Study the drawing (mm; zero at the part's minimum x, y, z) and answer. Round coordinates to 2 decimals unless told otherwise and drop trailing zeros. Order: outer loops, then holes, each group sorted by start corner. A loop starts at its lowest first (then second) coordinate and runs counter-clockwise, first axis right, second up. Notation, with made-up numbers: (-4, -18.75) - (5, -18.75) arc R32 ccw to (5, 7.25) - close; hole circle Ø10 at (-23, 70). An arc over 180 degrees is marked (long way). Use one line per item in the form item = value. Start each with the question number.
Q1. The part is cut by section B-B on y = 0.6. Determine the outline of the cut face in (x, z) (1 decimal).
Q2. The part is cut by section D-D on z = 14. Determine the outline of the cut face in (x, y) (1 decimal).
Q3. The part is cut by section C-C on x = 62.5. Determine the outline of the cut face in (y, z), plus the area to 3 significant figures.
Q4. Find the intervals of material crossed by line 1 (Z direction, x = 41, y = 0.9); line 2 (X direction, y = 1.7, z = 30) (1 decimal); line 3 (X direction, y = 0.45, z = 26) (1 decimal), in increasing order. Write a range as [from, to].
Q5. The part is cut by section A-A on z = 32.5. Determine the outline of the cut face in (x, y) (1 decimal), plus the area to 3 significant figures.
Q6. Given P1, Ø1, axis at y = 1, z = 20.5, coming from the +X side (1 decimal), flat-ended and moving along its own axis, determine where the tip first touches the part or whether it passes through.
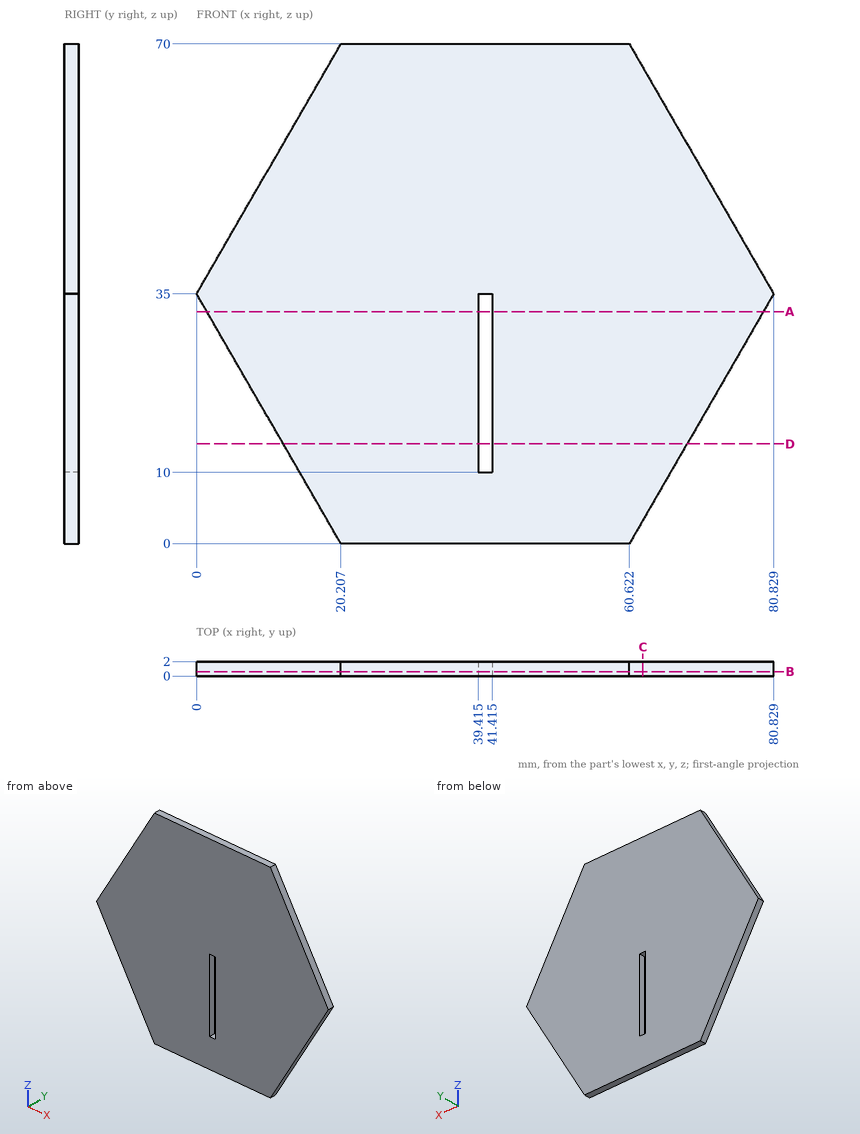
Found:
q1.outline = (0, 35) - (20.2, 0) - (60.6, 0) - (80.8, 35) - (60.6, 70) - (20.2, 70) - close; hole (39.4, 10) - (41.4, 10) - (41.4, 35) - (39.4, 35) - close
q2.outline = (12.1, 0) - (39.4, 0) - (39.4, 2) - (12.1, 2) - close; (41.4, 0) - (68.7, 0) - (68.7, 2) - (41.4, 2) - close
q3.outline = (0, 3.25) - (2, 3.25) - (2, 66.75) - (0, 66.75) - close
q3.area = 127 mm²
q4.line_1 = [0, 10], [35, 70]
q4.line_2 = [2.9, 39.4], [41.4, 77.9]
q4.line_3 = [5.2, 39.4], [41.4, 75.6]
q5.outline = (1.4, 0) - (39.4, 0) - (39.4, 2) - (1.4, 2) - close; (41.4, 0) - (79.4, 0) - (79.4, 2) - (41.4, 2) - close
q5.area = 152 mm²
q6.P1 = 72.7
